For this review, take the finished solid that the model builds, in its own axes (mm). A direction names the side the tool comes from. Round coordinates to 2 decimals unless told otherwise and drop trailing zeros. Write each loop counter-clockwise with the first axis right and the second up, starting at its lowest first coordinate (ties: lowest second). Pieces come first, ordered by that corner, then holes. Notation, with made-up numbers: (57, -30) -> (85, -30) arc R31 ccw to (85, 3) -> close; hole circle Ø8 at (81, 89.5). An arc over 180 degrees is marked (long way). Answer as CSV lines item,"result". Start each with the question number.
Item 1: For pin 1 Ø5 at (y, z) = (-60, 27.25) entering from +X; pin 2 Ø6 at (x, z) = (46.5, -14.5) entering from -Y, all flat-tipped, find the tip position at first contact; note any pin that passes through.
Item 2: Take a section at B-B on x = 4. Give the boundary of the cut face in (y, z), then the cut area to 3 significant figures.
Item 3: Machinability: for faces 1 (the flat face through (1, 0, -9)), 2 (the flat face through (-23, 1, 37.25)), which of the approach directions +Z, -Z, +X, -X, +Y, -Y give a long, thin tool a straight path to every point of the face, cutting with its end or side? Answer none if there is none.
Item 4: Mouldability with a two-part tool opening along X and no side actions: class faces 3 (the cylindrical face through (-72.465, -58.017, -26.99)), 4 (the cylindrical face through (-31.01, 2.54, 2.3)), 5 (the cylindrical face through (54.815, 2.535, 8.324)), 6 (the flat face through (-70, -35, -1)) as +X half, -X half, draft (parallel to the pull), parting line (faces both ways), or undercut.
Item 5: Wall thickness on probe 1 along X at (y, z) = (3, 0); probe 2 along Y at (x, z) = (-73, 27); probe 3 along Z at (x, y) = (-36.55, 2.1): over which ranges is each line inside the solid? List them lowest first. Write a range as from..to.
Item 6: Take a section at A-A on y = -60. Give the boundary of the cut face in (x, z), then the cut area to 4 significant figures.
Item 7: Take a section at D-D on y = -26.5. Give the boundary of the cut face in (x, z), then the cut area to 4 significant figures.
Item 8: Take a section at C-C on z = -23. Give the boundary of the cut face in (x, y), then the cut area to 3 significant figures.
```python
from build123d import *

# Parameters (mm, degrees)
CROQUIS1_W              = 150
CROQUIS1_H              = 74.5
SALIENTE_EXTRUIR1_DEPTH = 5
CROQUIS2_W              = 5
CROQUIS2_H              = 74.5
SALIENTE_EXTRUIR2_DEPTH = 70
CROQUIS3_R              = 2
CORTAR_EXTRUIR1_DEPTH   = 70
CROQUIS4_R              = 6
CROQUIS4_R_2            = 4.5
CROQUIS4_R_3            = 1.5
CORTAR_EXTRUIR2_DEPTH   = 70


with BuildPart() as part:
    # Croquis1 → Saliente-Extruir1 (new body)
    with BuildSketch(Plane(origin=(0, 0, 0), x_dir=(1, 0, 0), z_dir=(0, 1, 0))):
        Rectangle(CROQUIS1_W, CROQUIS1_H)
    extrude(amount=SALIENTE_EXTRUIR1_DEPTH)

    # Croquis2 → Saliente-Extruir2 (add)
    with BuildSketch(Plane.XZ):
        with Locations((-72.5, 0)):
            Rectangle(CROQUIS2_W, CROQUIS2_H)
    extrude(amount=SALIENTE_EXTRUIR2_DEPTH)

    # Croquis3 → Cortar-Extruir1 (cut)
    with BuildSketch(Plane(origin=(-70, 0, 0), x_dir=(0, 0, -1), z_dir=(1, 0, 0))):
        with Locations((-27.25, -10)):
            Circle(CROQUIS3_R)
        with Locations((27.25, -10)):
            Circle(CROQUIS3_R)
        with Locations((27.25, -60)):
            Circle(CROQUIS3_R)
        with Locations((-27.25, -60)):
            Circle(CROQUIS3_R)
    extrude(amount=-CORTAR_EXTRUIR1_DEPTH, mode=Mode.SUBTRACT)

    # Croquis4 → Cortar-Extruir2 (cut)
    with BuildSketch(Plane(origin=(0, 5, 0), x_dir=(1, 0, 0), z_dir=(0, 1, 0))):
        with Locations((-36.55, 0)):
            Circle(CROQUIS4_R)
        with Locations((53.45, -0.25)):
            Circle(CROQUIS4_R_2)
        with Locations((53.45, 7.25)):
            Circle(CROQUIS4_R_3)
        with Locations((53.429166747, -7.749971065)):
            Circle(CROQUIS4_R_3)
        with Locations((3.44984568, -0.111110682)):
            Circle(CROQUIS4_R)
    extrude(amount=-CORTAR_EXTRUIR2_DEPTH, mode=Mode.SUBTRACT)


solid = part.part
```
Output values:
1,pin 1,"stops at x = -70"
1,pin 2,"stops at y = 0"
2,outline,"(0, -37.25) -> (5, -37.25) -> (5, -5.86) -> (0, -5.86) -> close; (0, 6.09) -> (5, 6.09) -> (5, 37.25) -> (0, 37.25) -> close"
2,area,"313 mm^2"
3,face 1,"+Z, -Z, +X, -Y"
3,face 2,"+Z, +X, -X, +Y, -Y"
4,face 3,"draft"
4,face 4,"undercut"
4,face 5,"undercut"
4,face 6,"+X half"
5,probe 1,"x = -75..-42.55, -30.55..-2.55, 9.45..48.96, 57.94..75"
5,probe 2,"y = -70..-61.98, -58.02..-11.98, -8.02..5"
5,probe 3,"z = -37.25..-6, 6..37.25"
6,outline,"(-75, -37.25) -> (-70, -37.25) -> (-70, -29.25) -> (-75, -29.25) -> close; (-75, -25.25) -> (-70, -25.25) -> (-70, 25.25) -> (-75, 25.25) -> close; (-75, 29.25) -> (-70, 29.25) -> (-70, 37.25) -> (-75, 37.25) -> close"
6,area,"332.5 mm^2"
7,outline,"(-75, -37.25) -> (-70, -37.25) -> (-70, 37.25) -> (-75, 37.25) -> close"
7,area,"372.5 mm^2"
8,outline,"(-75, -70) -> (-70, -70) -> (-70, 0) -> (75, 0) -> (75, 5) -> (-75, 5) -> close"
8,area,"1,100 mm^2"
